from build123d import *
from OCP.BRepFilletAPI import BRepFilletAPI_MakeChamfer

# Parameters (mm, degrees)
SKETCH1_W               = 57.15
SKETCH1_H               = 30
BOSS_EXTRUDE1_DEPTH     = 11.6
SKETCH2_W               = 54
SKETCH2_H               = 21
CUT_EXTRUDE1_DEPTH      = 10.9
SKETCH3_R               = 5.375
CUT_EXTRUDE2_DEPTH      = 0.65
FILLET1_R               = 5
CUT_EXTRUDE3_DEPTH      = 66.467740147
CUT_EXTRUDE3_DEPTH_BACK = 1.35
SKETCH5_R               = 6.55
CHAMFER1_SIZE           = 5
CHAMFER1_SIZE2          = 8.660254038
FILLET2_R               = 2
SKETCH8_R               = 1.5
CUT_EXTRUDE5_DEPTH      = 10
SKETCH9_R               = 3
CUT_EXTRUDE6_DEPTH      = 1


with BuildPart() as part:
    # Sketch1 → Boss-Extrude1 (new body)
    with BuildSketch(Plane(origin=(0, 0, 0), x_dir=(1, 0, 0), z_dir=(0, 1, 0))):
        with Locations((28.575, 15)):
            Rectangle(SKETCH1_W, SKETCH1_H)
    extrude(amount=BOSS_EXTRUDE1_DEPTH)

    # Sketch2 → Cut-Extrude1 (cut)
    with BuildSketch(Plane(origin=(0, 0, 0), x_dir=(-1, 0, 0), z_dir=(0, -1, 0))):
        with Locations((-28.575, 15)):
            Rectangle(SKETCH2_W, SKETCH2_H)
    extrude(amount=-CUT_EXTRUDE1_DEPTH, mode=Mode.SUBTRACT)

    # Sketch3 → Cut-Extrude2 (cut)
    with BuildSketch(Plane(origin=(0, 11.6, 0), x_dir=(1, 0, 0), z_dir=(0, 1, 0))):
        with Locations(Location((17.58, 15, 0), (0, 0, 270))):
            Circle(SKETCH3_R)
    extrude(amount=-CUT_EXTRUDE2_DEPTH, mode=Mode.SUBTRACT)

    # Fillet1
    fillet1_edges = [part.edges().sort_by_distance(p)[0] for p in [
        (0, 5.8, -30),
        (0, 5.8, 0),
    ]]
    fillet(fillet1_edges, radius=FILLET1_R)

    # Sketch5 → Cut-Extrude3 (cut, two sides: drawn at the far end of the back side and taken through both)
    with BuildSketch(Plane(origin=(0, 10.95, 0), x_dir=(1, 0, 0), z_dir=(0, 1, 0)).offset(-CUT_EXTRUDE3_DEPTH_BACK)):
        with Locations(Location((18.475, 15, 0), (0, 0, 90))):
            Circle(SKETCH5_R)
    extrude(amount=CUT_EXTRUDE3_DEPTH + CUT_EXTRUDE3_DEPTH_BACK, mode=Mode.SUBTRACT)

    # Chamfer1: one chamfer whose edges measure the first distance from different faces: ONE call of the kernel's chamfer builder (chamfer() names one face for all edges)
    chamfer1_edges_1 = [part.edges().sort_by_distance(p)[0] for p in [
        (1.575, 10.9, -15),
    ]]
    chamfer1_side_1 = [part.faces().sort_by_distance(p)[0] for p in [
        (1.575, 5.45, -15),
    ]]
    chamfer1_edges_2 = [part.edges().sort_by_distance(p)[0] for p in [
        (55.575, 10.9, -15),
    ]]
    chamfer1_side_2 = [part.faces().sort_by_distance(p)[0] for p in [
        (55.575, 5.45, -15),
    ]]
    chamfer1 = BRepFilletAPI_MakeChamfer(part.part.solid().wrapped)
    for e in chamfer1_edges_1:
        chamfer1.Add(CHAMFER1_SIZE, CHAMFER1_SIZE2, e.wrapped, chamfer1_side_1[0].wrapped)  # the first distance lies on this face
    for e in chamfer1_edges_2:
        chamfer1.Add(CHAMFER1_SIZE, CHAMFER1_SIZE2, e.wrapped, chamfer1_side_2[0].wrapped)  # the first distance lies on this face
    add(Compound.cast(chamfer1.Shape()), mode=Mode.REPLACE)

    # Fillet2
    fillet2_edges = [part.edges().sort_by_distance(p)[0] for p in [
        (57.15, 11.6, -15),
        (31.075, 11.6, -30),
        (0, 11.6, -15),
        (31.075, 11.6, 0),
        (1.464466094, 11.6, -1.464466094),
        (1.464466094, 11.6, -28.535533906),
        (57.15, 5.8, -30),
        (57.15, 5.8, 0),
    ]]
    fillet(fillet2_edges, radius=FILLET2_R)

    # Sketch8 → Cut-Extrude5 (cut)
    with BuildSketch(Plane(origin=(0, 11.6, 0), x_dir=(1, 0, 0), z_dir=(0, 1, 0))):
        with Locations(Location((52.475, 20, 0), (0, 0, 270))):
            Circle(SKETCH8_R)
        with Locations(Location((52.475, 10, 0), (0, 0, 270))):
            Circle(SKETCH8_R)
        with Locations(Location((4.475, 20, 0), (0, 0, 270))):
            Circle(SKETCH8_R)
        with Locations(Location((4.475, 10, 0), (0, 0, 270))):
            Circle(SKETCH8_R)
    extrude(amount=-CUT_EXTRUDE5_DEPTH, mode=Mode.SUBTRACT)

    # Sketch9 → Cut-Extrude6 (cut)
    with BuildSketch(Plane(origin=(0, 11.6, 0), x_dir=(1, 0, 0), z_dir=(0, 1, 0))):
        with Locations(Location((4.475, 20, 0), (0, 0, 270))):
            Circle(SKETCH9_R)
        with Locations(Location((4.475, 10, 0), (0, 0, 270))):
            Circle(SKETCH9_R)
        with Locations(Location((52.475, 10, 0), (0, 0, 270))):
            Circle(SKETCH9_R)
        with Locations(Location((52.475, 20, 0), (0, 0, 270))):
            Circle(SKETCH9_R)
    extrude(amount=-CUT_EXTRUDE6_DEPTH, mode=Mode.SUBTRACT)


solid = part.part
Could you check a few things on this model? Use its own coordinates, in mm. A direction names the side the tool comes from. Round coordinates to 2 decimals unless told otherwise and drop trailing zeros. Loops run counter-clockwise (first coordinate to the right, second up) from the corner with the lowest first, then second, coordinate; pieces in that order, holes last. Notation, with made-up numbers: (-18, -30.75) - (21, -30.75) arc R21 ccw to (21, -5.75) - close; hole circle Ø9 at (18.25, 5.5). An arc over 180 degrees is marked (long way). Write item = value, one per line.
1) Imagine slicing it at A-A (z = -15). Please give me the cut outline in (x, y) (3 decimals).
Computed:
outline = (0, 0) - (1.575, 0) - (1.575, 5.9) - (10.235, 10.9) - (11.925, 10.9) - (11.925, 11.6) - (2, 11.6) arc R2 ccw to (0, 9.6) - close; (25.025, 10.9) - (46.915, 10.9) - (55.575, 5.9) - (55.575, 0) - (57.15, 0) - (57.15, 9.6) arc R2 ccw to (55.15, 11.6) - (25.025, 11.6) - close
2) If we mould it in two halves opening along Z, with no side actions, what happens to faces 1 (the cylindrical face through (1, 5, -2)), 2 (the cylindrical face through (54.503, 11.107, -12.211)), 3 (the flat face through (29, 5, -25.5)), 4 (the cylindrical face through (0.57, 11, -15.14))? For each: pulls with the +Z half, pulls with the -Z half, needs draft (parallel to the pull), parting line crosses it, or undercut.
Computed:
face_1 = pulls with the +Z half
face_2 = undercut
face_3 = undercut
face_4 = needs draft
3) I need wall thicknesses on line 1 along Z through (x, y) = (18, 6.5); line 2 along X through (y, z) = (5, -7.75) (3 decimals); line 3 along Z through (x, y) = (7, 11). Which ranges of each line are inside material? Lowest first, please. Write a range as from..to.
Computed:
line_1 = -30..-25.5, -4.5..0
line_2 = 0..1.575, 55.575..57.15
line_3 = -29.43..-21.62, -18.38..-11.62, -8.38..-0.57
4) I'm going to push flat-ended pins straight in: P1, Ø10.5, axis at x = 22.5, z = -13, coming from the -Y side; P2, Ø3.5, axis at x = 52.475, z = -20, coming from the +Y side; P3, Ø5.5, axis at x = 52.475, z = -10, coming from the -Y side. Where does each tip first touch, or does it pass through?
Computed:
P1 = 10.9
P2 = 10.6
P3 = 6.1
5) Imagine slicing it at C-C (z = -10.25). Give the number of separate pieces and of enclosed holes in the cut face, and give its area (3 significant figures).
Computed:
separate_pieces = 4
enclosed_holes = 0
area = 80.1 mm2
6) Imagine slicing it at D-D (x = 19). Please give me the cut outline in (y, z).
Computed:
outline = (0, -30) - (9.6, -30) arc R2 ccw to (11.6, -28) - (11.6, -21.53) - (10.9, -21.53) - (10.9, -25.5) - (0, -25.5) - close; (0, -4.5) - (10.9, -4.5) - (10.9, -8.47) - (11.6, -8.47) - (11.6, -2) arc R2 ccw to (9.6, 0) - (0, 0) - close
7) Imagine slicing it at B-B (x = 28). Please give me the cut outline in (y, z), and give its area (3 significant figures).
Computed:
outline = (0, -30) - (9.6, -30) arc R2 ccw to (11.6, -28) - (11.6, -2) arc R2 ccw to (9.6, 0) - (0, 0) - (0, -4.5) - (10.9, -4.5) - (10.9, -25.5) - (0, -25.5) - close
area = 117 mm2
8) On a 3-axis mill with a long thin cutter (end or side, diameter ignored), from which of +Z, -Z, +X, -X, +Y, -Y can I reach the whole of each face in a straight line? I mean faces 5 (the flat face through (29, 5, -4.5)), 6 (the cylindrical face through (1, 5, -28)), 7 (the flat face through (54, 10.6, -19)). Say none if no direction works.
Computed:
face_5 = -Y
face_6 = -Z, -X, +Y, -Y
face_7 = +Y
